from build123d import *

# Parameters (mm, degrees)
CIRPATTERN1_COUNT  = 8
SKETCH9_R          = 56.881527661
SKETCH9_R_2        = 53.881527661
CUT_EXTRUDE1_DEPTH = 6


with BuildPart() as part:
    # Sketch1 → Revolve2 (revolve)
    with BuildSketch(Plane.XY, mode=Mode.PRIVATE) as revolve2_sk:
        with BuildLine():
            Line((71.727523602, 109.927507641), (76.490023602, 109.927507641))
            Line((76.490023602, 109.927507641), (76.490023602, -212.127513222))
            Line((76.490023602, -212.127513222), (53.881527661, -212.127513222))
            Line((53.881527661, -212.127513222), (53.881527661, -59.727513222))
            add(Edge.make_bspline(
                [(53.881527661, -59.727513222), (53.88152643, -59.656983157), (53.880997287, -59.515406103), (53.878621437, -59.181564616), (53.872296838, -58.904795493), (53.862811351, -58.532567488), (53.850168453, -58.212837622), (53.830417626, -57.781594443), (53.800405285, -57.280959899), (53.756193121, -56.687998165), (53.677288452, -55.848480366), (53.577426861, -55.00816586), (53.456675786, -54.17243543), (53.286810822, -53.17242524), (53.092064187, -52.177442821), (52.86637512, -51.188539083), (52.610014224, -50.207489038), (52.32928934, -49.23307774), (52.024348739, -48.265969224), (51.633537831, -47.149135067), (51.139520361, -45.890408405), (50.598733753, -44.650968804), (50.012060928, -43.432701526), (49.380120231, -42.237093239), (48.704125229, -41.066154879), (47.98447552, -39.920972657), (47.223102138, -38.804076239), (46.51986906, -37.851451785), (45.893537937, -37.055672123), (45.352817681, -36.403381282), (44.915126948, -35.894247633), (44.51477619, -35.446992657), (44.181457503, -35.084631185), (43.873924624, -34.760340151), (43.674072407, -34.551549451), (43.444392073, -34.318516288), (43.343783151, -34.217162055), (43.293911001, -34.167289665)],
                knots=[0.082637729, 0.082637729, 0.082637729, 0.082637729, 0.082637729, 0.092574926, 0.102512123, 0.11244932, 0.122386517, 0.132323714, 0.142260911, 0.162135305, 0.182009699, 0.201884093, 0.24163288, 0.261507274, 0.281381668, 0.321130456, 0.360879243, 0.380753637, 0.400628031, 0.440376819, 0.480125606, 0.519874394, 0.559623181, 0.599371969, 0.639120757, 0.678869544, 0.718618332, 0.75836712, 0.798115907, 0.817990301, 0.837864695, 0.857739089, 0.877613483, 0.88755068, 0.897487877, 0.907425074, 0.91736227, 0.91736227, 0.91736227, 0.91736227, 0.91736227], degree=4))
            Line((43.293911001, -34.167289665), (34.686282803, -25.559661468))
            add(Edge.make_bspline(
                [(24.099067874, 0.000160672), (24.099069105, -0.070367974), (24.099598252, -0.213423516), (24.101973937, -0.543022243), (24.108298331, -0.823999723), (24.117783452, -1.194661398), (24.130425744, -1.513274385), (24.146225968, -1.86177893), (24.165181227, -2.193546198), (24.19281884, -2.617908727), (24.232287047, -3.121873274), (24.303299707, -3.879818002), (24.423126678, -4.886289715), (24.599486044, -6.056550088), (24.850885233, -7.385005743), (25.151795313, -8.703413843), (25.501770623, -10.009476538), (25.900360983, -11.301658927), (26.346945392, -12.577938667), (26.841003323, -13.836726817), (27.381673122, -15.076036463), (27.968479386, -16.294449129), (28.600139398, -17.489778131), (29.276532396, -18.661127095), (29.995445102, -19.805582737), (30.758021999, -20.923699417), (31.459167193, -21.874251104), (32.088736123, -22.673284825), (32.624128416, -23.320261484), (33.072255768, -23.839844364), (33.508450026, -24.329655594), (33.935826121, -24.788323739), (34.24555864, -25.11370766), (34.536859958, -25.409488397), (34.636412425, -25.509789283), (34.686282803, -25.559661468)],
                knots=[0.082637729, 0.082637729, 0.082637729, 0.082637729, 0.082637729, 0.092574926, 0.102512123, 0.11244932, 0.122386517, 0.132323714, 0.142260911, 0.152198108, 0.162135305, 0.182009699, 0.201884093, 0.24163288, 0.281381668, 0.321130456, 0.360879243, 0.400628031, 0.440376819, 0.480125606, 0.519874394, 0.559623181, 0.599371969, 0.639120757, 0.678869544, 0.718618332, 0.75836712, 0.798115907, 0.817990301, 0.837864695, 0.857739089, 0.877613483, 0.897487877, 0.907425074, 0.91736227, 0.91736227, 0.91736227, 0.91736227, 0.91736227], degree=4))
            add(Edge.make_bspline(
                [(24.099067874, 0.000160672), (24.0990685, 0.036053324), (24.099606331, 0.110274362), (24.102023723, 0.267801742), (24.108461568, 0.427224789), (24.120533599, 0.646924939), (24.141435087, 0.901594), (24.175184719, 1.202697945), (24.226499305, 1.54221117), (24.290543701, 1.881157449), (24.367141601, 2.216515092), (24.456323571, 2.549400093), (24.557741413, 2.878253317), (24.671619071, 3.203507713), (24.797196771, 3.523787829), (24.935285977, 3.839827405), (25.084070301, 4.149442857), (25.246012222, 4.454943795), (25.416488505, 4.751462248), (25.602514721, 5.045864533), (25.79178827, 5.325679608), (26.004405474, 5.610888215), (26.178876374, 5.83307432), (26.366345756, 6.050112309), (26.504555248, 6.208802318), (26.67044207, 6.382282451), (26.744520261, 6.458639514), (26.795279203, 6.509400323)],
                knots=[0.082568816, 0.082568816, 0.082568816, 0.082568816, 0.082568816, 0.102426634, 0.122284453, 0.142142271, 0.162000089, 0.201715725, 0.241431362, 0.281146998, 0.320862634, 0.360578271, 0.400293907, 0.440009544, 0.47972518, 0.519440816, 0.559156453, 0.598872089, 0.638587725, 0.678303362, 0.718018998, 0.757734635, 0.797450271, 0.837165907, 0.857023726, 0.876881544, 0.91659718, 0.91659718, 0.91659718, 0.91659718, 0.91659718], degree=4))
            add(Edge.make_bspline(
                [(26.795279203, 6.509400323), (49.261401403, 34.636114842), (71.727523602, 109.927507641)],
                knots=[0, 0, 0, 1, 1, 1], degree=2))
        make_face()
    revolve(revolve2_sk.sketch.rotate(Axis((-0.005532126, 165.815985114, 0), (0, -1, 0)), 180), axis=Axis((-0.005532126, 165.815985114, 0), (0, -1, 0)))

    # Sketch4 → 3/8-24 Tapped Hole1 (revolve, cut)
    with BuildSketch(Plane(origin=(65.2, -212.127513222, 0), x_dir=(0, 0, -1), z_dir=(1, 0, 0))):
        Polygon((0, 0), (0, 27.533468714), (4.2164, 25), (4.2164, 0), align=None)
    f_3_8_24_tapped_hole1 = revolve(axis=Axis((65.2, -218.477513222, 0), (0, 1, 0)), mode=Mode.SUBTRACT)

    # CirPattern1: 3/8-24 Tapped Hole1 ×8 about axis
    cirpattern1_axis = Axis((0, -228.487022387, 0), (-1.634718801334702e-05, 0.9999999998663848, 0))
    for i in range(1, CIRPATTERN1_COUNT):
        add(f_3_8_24_tapped_hole1.rotate(cirpattern1_axis, i * 360 / CIRPATTERN1_COUNT), mode=Mode.SUBTRACT)

    # Sketch9 → Cut-Extrude1 (cut)
    with BuildSketch(Plane.XZ.offset(212.127513222)):
        Circle(SKETCH9_R)
        Circle(SKETCH9_R_2, mode=Mode.SUBTRACT)
    extrude(amount=-CUT_EXTRUDE1_DEPTH, mode=Mode.SUBTRACT)


with BuildPart() as cut_extrude1_kept_piece:
    # of the separate pieces the step leaves, the one the design keeps (cut_extrude1_pieces_kept)
    add(part.part.solids().sort_by_distance((-71.738587854, 109.927507641, 0))[0])


solid = cut_extrude1_kept_piece.part
Geometry check sheet. Reference: the model listing, model coordinates, mm. Give positions to 0.01 mm unless a question says otherwise; leave off trailing zeros.
1) Draft check along Z on faces 1 (the cylindrical face through (69.316, -199.803, 0.914)), 2 (the flat face through (12, -212.128, 56)), 3 (the cylindrical face through (9.953, -53.354, -75.845)). Enter one of: released by +Z, released by -Z, zero draft, split by the parting line, or undercut.
Results are:
face 1: undercut
face 2: zero draft
face 3: split by the parting line
2) Material ranges on probe 1 along Z at (x, y) = (0, -207); probe 2 along Z at (x, y) = (17, -59); probe 3 along X at (y, z) = (-135.5, 18.5), recorded low to high.
Results are:
probe 1: z = -76.5 to -69.42, -60.98 to -56.88, 56.88 to 60.98, 69.42 to 76.5
probe 2: z = -74.58 to -51.13, 51.13 to 74.58
probe 3: x = -74.23 to -50.62, 50.61 to 74.22
3) Gauge pin test, flat ends, axial feed: pin 1 (1 mm diameter, centred on y = -58.5, z = 2.5, fed in from -X); pin 2 (1.5 mm diameter, centred on y = -1, z = -19, fed in from -X); pin 3 (4 mm diameter, centred on x = -4.5, y = 27.5, fed in from -Z). Record the tip position at first contact, or that the pin passes through.
Results are:
pin 1: stops at x = -76.47
pin 2: stops at x = -74.29
pin 3: stops at z = -76.45
